Check sheet for the modelled part. Datum: model origin and axes. Units: mm. Round coordinates to 2 decimals unless told otherwise and drop trailing zeros. Order: outer loops, then holes, each group sorted by start corner. A loop starts at its lowest first (then second) coordinate and runs counter-clockwise, first axis right, second up. Notation, with made-up numbers: M -7,20 L 25,20 A28 cw 25,59 Z; hole C 89,73.25 d5. An arc over 180 degrees is marked long. One line per item, written item: value. Start each with the question number.
(1) Cross-section at A-A, the plane z = 4. Enter the section's corners in (x, y).
(2) Thickness scan on L1, parallel to Y at x = -199.5, z = 6.25; L2, parallel to X at y = 5.5, z = 6.25; L3, parallel to X at y = 2, z = 2. Record the ranges inside material, lowest first.
(3) Depth check by flat-ended pin: pin 1 Ø0.8 at (y, z) = (16, 2) entering from -X; pin 2 Ø4 at (x, z) = (-174, 1.5) entering from -Y; pin 3 Ø1 at (y, z) = (-2, 1.5) entering from -X. Enter the tip coordinate at first touch or a pass-through.
(4) Cross-section at B-B, the plane x = -4. Enter the section's corners in (y, z).
(5) Cross-section at C-C, the plane x = -139. Enter the section's corners in (y, z), and give its area (3 significant figures).
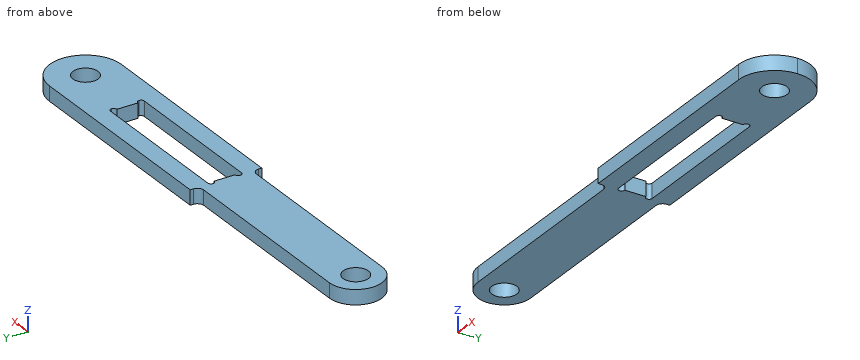
from build123d import *

# Parameters (mm, degrees)
F0_R     = 6
F1_DEPTH = 7
F3_DEPTH = 7.001
F4_R     = 3


with BuildPart() as f1:
    # F0 (on Top) → F1 (new body)
    with BuildSketch(Plane.XY):
        with BuildLine():
            ThreePointArc((0, -17), (-17, 0), (0, 17))
            Line((0, 17), (-104, 17))
            Line((-104, 17), (-104, 12.5))
            Line((-104, 12.5), (-200, 12.5))
            ThreePointArc((-200, 12.5), (-191.1611652352, 8.8388347648), (-187.5, 0))
            ThreePointArc((-187.5, 0), (-191.1611652352, -8.8388347648), (-200, -12.5))
            Line((-200, -12.5), (-104, -12.5))
            Line((-104, -12.5), (-104, -17))
            Line((-104, -17), (0, -17))
        make_face()
        with BuildLine():
            ThreePointArc((0, -17), (12.0208152802, -12.0208152802), (17, 0))
            ThreePointArc((17, 0), (12.0208152802, 12.0208152802), (0, 17))
            ThreePointArc((0, 17), (-17, 0), (0, -17))
        make_face()
        Circle(F0_R, mode=Mode.SUBTRACT)
        with BuildLine():
            ThreePointArc((-187.5, 0), (-191.1611652352, 8.8388347648), (-200, 12.5))
            ThreePointArc((-200, 12.5), (-212.5, 0), (-200, -12.5))
            ThreePointArc((-200, -12.5), (-191.1611652352, -8.8388347648), (-187.5, 0))
        make_face()
        with Locations((-200, 0)):
            Circle(F0_R, mode=Mode.SUBTRACT)
    extrude(amount=F1_DEPTH)

    # F2 (on face) → F3 (cut, through all)
    with BuildSketch(Plane.XY.offset(7)):
        with BuildLine():
            ThreePointArc((-31, 5), (-32.5, 6.5), (-31, 8))
            Line((-31, 8), (-103, 8))
            ThreePointArc((-103, 8), (-101.9393398282, 7.5606601718), (-101.5, 6.5))
            ThreePointArc((-101.5, 6.5), (-101.9393398282, 5.4393398282), (-103, 5))
            Line((-103, 5), (-103, -5))
            ThreePointArc((-103, -5), (-101.9393398282, -5.4393398282), (-101.5, -6.5))
            ThreePointArc((-101.5, -6.5), (-101.9393398282, -7.5606601718), (-103, -8))
            Line((-103, -8), (-31, -8))
            ThreePointArc((-31, -8), (-32.5, -6.5), (-31, -5))
            Line((-31, -5), (-31, 5))
        make_face()
        with BuildLine():
            ThreePointArc((-29.5, 6.5), (-29.9393398282, 7.5606601718), (-31, 8))
            Line((-31, 8), (-31, 5))
            ThreePointArc((-31, 5), (-29.9393398282, 5.4393398282), (-29.5, 6.5))
        make_face()
        with BuildLine():
            Line((-31, 5), (-31, 8))
            ThreePointArc((-31, 8), (-32.5, 6.5), (-31, 5))
        make_face()
        with BuildLine():
            ThreePointArc((-101.5, 6.5), (-101.9393398282, 7.5606601718), (-103, 8))
            Line((-103, 8), (-103, 5))
            ThreePointArc((-103, 5), (-101.9393398282, 5.4393398282), (-101.5, 6.5))
        make_face()
        with BuildLine():
            Line((-103, 5), (-103, 8))
            ThreePointArc((-103, 8), (-104.5, 6.5), (-103, 5))
        make_face()
        with BuildLine():
            ThreePointArc((-29.5, -6.5), (-29.9393398282, -5.4393398282), (-31, -5))
            Line((-31, -5), (-31, -8))
            ThreePointArc((-31, -8), (-29.9393398282, -7.5606601718), (-29.5, -6.5))
        make_face()
        with BuildLine():
            Line((-31, -8), (-31, -5))
            ThreePointArc((-31, -5), (-32.5, -6.5), (-31, -8))
        make_face()
        with BuildLine():
            ThreePointArc((-101.5, -6.5), (-101.9393398282, -5.4393398282), (-103, -5))
            Line((-103, -5), (-103, -8))
            ThreePointArc((-103, -8), (-101.9393398282, -7.5606601718), (-101.5, -6.5))
        make_face()
        with BuildLine():
            Line((-103, -8), (-103, -5))
            ThreePointArc((-103, -5), (-104.5, -6.5), (-103, -8))
        make_face()
    extrude(amount=-F3_DEPTH, mode=Mode.SUBTRACT)

    # F4
    f4_edges = [f1.edges().sort_by_distance(p)[0] for p in [
        (-104, 12.5, 3.5),
        (-104, -12.5, 3.5),
    ]]
    fillet(f4_edges, radius=F4_R)


solid = f1.part
Values found:
1. outline: M -200,-12.5 L -107,-12.5 A3 cw -104,-15.5 L -104,-17 L 0,-17 A17 ccw 0,17 L -104,17 L -104,15.5 A3 cw -107,12.5 L -200,12.5 A12.5 ccw Z; hole C -200,0 d12; hole M -103,-8 L -31,-8 A1.5 ccw -31,-5 L -31,5 A1.5 ccw -31,8 L -103,8 A1.5 ccw -103,5 L -103,-5 A1.5 ccw Z; hole C 0,0 d12
2. L1: -12.5 to -5.98, 5.98 to 12.5
2. L2: -211.22 to -202.4, -197.6 to -104.12, -29.88 to -2.4, 2.4 to 16.09
2. L3: -212.34 to -205.66, -194.34 to -103, -31 to -5.66, 5.66 to 16.88
3. pin 1: x = -104
3. pin 2: y = -12.5
3. pin 3: x = -212.41
4. outline: M -17,0 L -4.47,0 L -4.47,7 L -17,7 Z; M 4.47,0 L 17,0 L 17,7 L 4.47,7 Z
5. outline: M -12.5,0 L 12.5,0 L 12.5,7 L -12.5,7 Z
5. area: 175 mm^2
